Geometry: final body of the model. Coordinates: model frame, mm. A direction names the side the tool comes from. Coordinates: 2 decimals unless noted, no trailing zeros. Loops run counter-clockwise (first coordinate to the right, second up) from the corner with the lowest first, then second, coordinate; pieces in that order, holes last. Notation, with made-up numbers: (32.5, -14) - (39.5, -14) arc R21 ccw to (39.5, -2) - close; hole circle Ø1 at (38, -10). An arc over 180 degrees is marked (long way). Answer in a Markdown table with one row per item.
from build123d import *

# Parameters (mm, degrees)
BOSS_EXTRUDE1_DEPTH = 10
SKETCH3_R           = 1.75
CUT_EXTRUDE1_DEPTH  = 10
SKETCH2_R           = 1.75
CUT_EXTRUDE2_DEPTH  = 10
FILLET1_R           = 2


with BuildPart() as part:
    # Sketch1 → Boss-Extrude1 (new body)
    with BuildSketch(Plane.XY):
        with BuildLine():
            Line((3.5, -17.05), (3.5, -10.481054336))
            ThreePointArc((3.5, -10.481054336), (11.008967033, 0.951391014), (1.65, 10.926115504))
            Line((1.65, 10.926115504), (1.65, 20.437453856))
            Line((1.65, 20.437453856), (1.65, 22.937453856))
            Line((1.65, 22.937453856), (7.65, 22.937453856))
            Line((7.65, 22.937453856), (7.65, 15.237453856))
            ThreePointArc((7.65, 15.237453856), (17.016334424, 1.070916786), (9.5, -14.158124876))
            Line((9.5, -14.158124876), (9.5, -21.858124876))
            Line((9.5, -21.858124876), (3.5, -21.858124876))
            Line((3.5, -21.858124876), (3.5, -19.358124876))
            Line((3.5, -19.358124876), (3.5, -17.05))
        make_face()
    extrude(amount=BOSS_EXTRUDE1_DEPTH)

    # Sketch3 → Cut-Extrude1 (cut)
    with BuildSketch(Plane(origin=(9.5, 0, 0), x_dir=(0, 0, -1), z_dir=(1, 0, 0))):
        with Locations(Location((-5, -18.008124876, 0), (0, 0, 90))):
            Circle(SKETCH3_R)
    extrude(amount=-CUT_EXTRUDE1_DEPTH, mode=Mode.SUBTRACT)

    # Sketch2 → Cut-Extrude2 (cut)
    with BuildSketch(Plane(origin=(7.65, 0, 0), x_dir=(0, 0, -1), z_dir=(1, 0, 0))):
        with Locations((-5, 19.087453856)):
            Circle(SKETCH2_R)
    extrude(amount=-CUT_EXTRUDE2_DEPTH, mode=Mode.SUBTRACT)

    # Fillet1
    fillet1_edges = [part.edges().sort_by_distance(p)[0] for p in [
        (4.65, 22.937453856, 0),
        (6.5, -21.858124876, 10),
        (6.5, -21.858124876, 0),
        (4.65, 22.937453856, 10),
    ]]
    fillet(fillet1_edges, radius=FILLET1_R)


solid = part.part
(1) Cut plane B-B on x = 8.5. Output: boundary loops of the cut face in (y, z).
Verdict:
| item | result |
|---|---|
| outline | (-21.86, 2) arc R2 ccw to (-19.86, 0) - (-7.06, 0) - (-7.06, 10) - (-19.86, 10) arc R2 ccw to (-21.86, 8) - close; (7.06, 0) - (14.78, 0) - (14.78, 10) - (7.06, 10) - close; hole circle Ø3.5 at (-18.01, 5) |
(2) First-contact query: pin 1 Ø6 at (y, z) = (-15.5, 3.5) entering from -X; pin 2 Ø1 at (x, z) = (9.5, 5) entering from +Y; pin 3 Ø3 at (x, y) = (8, 17) entering from -Z; pin 4 Ø3 at (y, z) = (19.09, 5) entering from -X. Flat tips, straight axial feed; report the tip coordinate or a pass-through.
Verdict:
| item | result |
|---|---|
| pin 1 | stops at x = 3.5 |
| pin 2 | stops at y = 14.48 |
| pin 3 | stops at z = 0 |
| pin 4 | passes through |
(3) Cut plane C-C on y = -19. Output: boundary loops of the cut face in (x, z), then the cut area to 3 significant figures.
Verdict:
| item | result |
|---|---|
| outline | (3.5, 0) - (9.5, 0) - (9.5, 3.56) - (3.5, 3.56) - close; (3.5, 6.44) - (9.5, 6.44) - (9.5, 10) - (3.5, 10) - close |
| area | 42.7 mm² |
(4) Pull-direction query (Z, two-part tool) for faces 5 (the face through (4.692, 18.023, 6.389)), 6 (the face through (6.54, -19.4, 3.94)), 7 (the face through (4.692, 22.336, 9.43)), 8 (the face through (7, -21.858, 5)); classes: pulls with the +Z half, pulls with the -Z half, needs draft (parallel to the pull), parting line crosses it, or undercut.
Verdict:
| item | result |
|---|---|
| face 5 | undercut |
| face 6 | undercut |
| face 7 | pulls with the +Z half |
| face 8 | needs draft |
(5) Ray query, probe 1 along Y at (x, z) = (4.25, 3.5); probe 2 along Y at (x, z) = (9, 2); probe 3 along X at (y, z) = (-14.5, 7.75). Return the intervals inside material, ascending.
Verdict:
| item | result |
|---|---|
| probe 1 | y = -21.86 to -18.91, -17.11 to -10.2, 10.2 to 18.19, 19.99 to 22.94 |
| probe 2 | y = -21.86 to -6.41, 6.41 to 14.48 |
| probe 3 | x = 3.5 to 9.5 |
(6) Access query for faces 1 (the face through (3.5, -16, 5)), 2 (the face through (7.65, 21, 5)), 3 (the face through (4.692, 22.336, 0.57)), 4 (the face through (9.5, -16, 5)). Directions: +Z, -Z, +X, -X, +Y, -Y. A direction counts if a zero-diameter tool reaches every point of the face in a straight line with its end or side. Return the directions, or none.
Verdict:
| item | result |
|---|---|
| face 1 | +Z, -Z, -X, -Y |
| face 2 | +Z, -Z, +X, +Y |
| face 3 | -Z, +X, -X, +Y |
| face 4 | +Z, -Z, +X, -Y |
(7) Cut plane A-A on z = 5. Output: boundary loops of the cut face in (x, y), then the cut area to 3 significant figures.
Verdict:
| item | result |
|---|---|
| outline | (1.65, 10.93) arc R11.05 cw to (3.5, -10.48) - (3.5, -16.26) - (9.5, -16.26) - (9.5, -14.16) arc R17.05 ccw to (7.65, 15.24) - (7.65, 17.34) - (1.65, 17.34) - close; (1.65, 20.84) - (7.65, 20.84) - (7.65, 22.94) - (1.65, 22.94) - close; (3.5, -21.86) - (9.5, -21.86) - (9.5, -19.76) - (3.5, -19.76) - close |
| area | 269 mm² |
(8) Cut plane D-D on y = 1. Output: boundary loops of the cut face in (x, z).
Verdict:
| item | result |
|---|---|
| outline | (11, 0) - (17.02, 0) - (17.02, 10) - (11, 10) - close |
